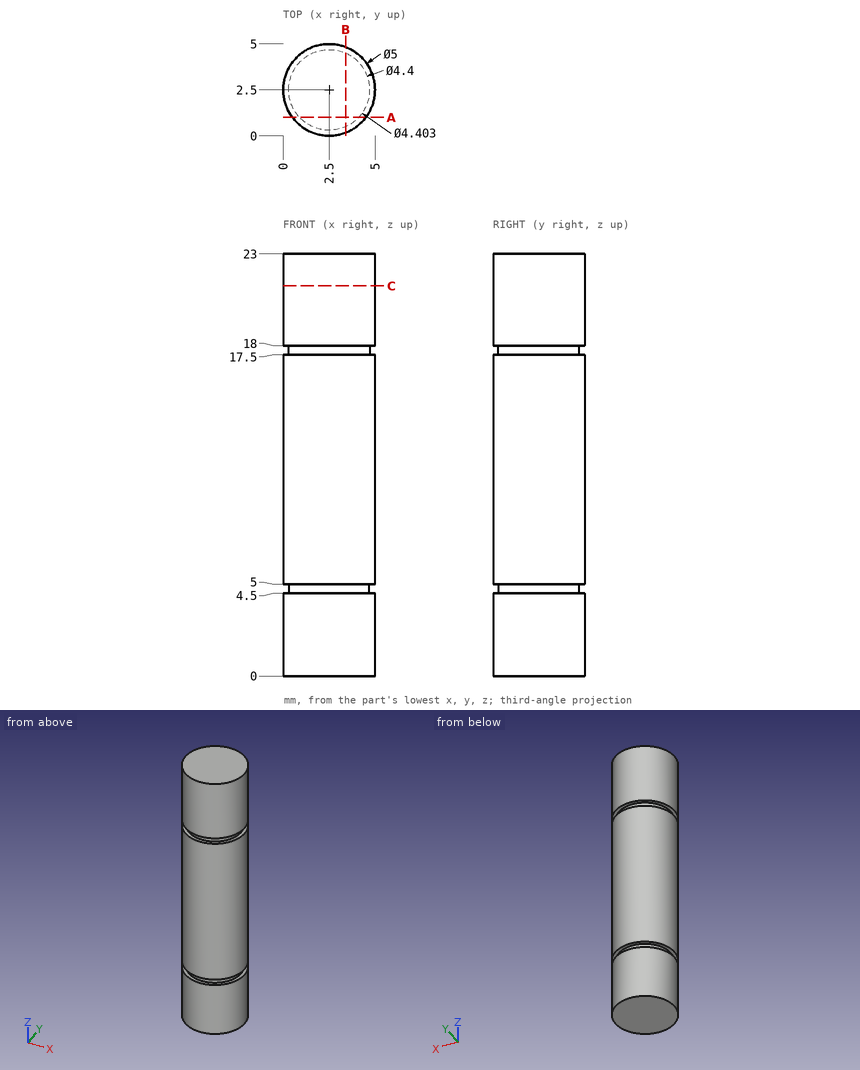
Print and shaded views of the part. All mm, measured from the part's lowest x, y and z. Round coordinates to 2 decimals unless told otherwise and drop trailing zeros. Write each loop counter-clockwise with the first axis right and the second up, starting at its lowest first coordinate (ties: lowest second). Pieces come first, ordered by that corner, then holes.
Item 1: Cut at B-B, the plane x = 3.4. Give the cut face in (y, z).
Results:
outline: (0.17, 0) - (4.83, 0) - (4.83, 4.5) - (4.51, 4.5) - (4.51, 5) - (4.83, 5) - (4.83, 17.5) - (4.51, 17.5) - (4.51, 18) - (4.83, 18) - (4.83, 23) - (0.17, 23) - (0.17, 18) - (0.49, 18) - (0.49, 17.5) - (0.17, 17.5) - (0.17, 5) - (0.49, 5) - (0.49, 4.5) - (0.17, 4.5) - close
Item 2: Cut at A-A, the plane y = 1. Give the cut face in (x, z).
Results:
outline: (0.5, 0) - (4.5, 0) - (4.5, 4.5) - (4.11, 4.5) - (4.11, 5) - (4.5, 5) - (4.5, 17.5) - (4.11, 17.5) - (4.11, 18) - (4.5, 18) - (4.5, 23) - (0.5, 23) - (0.5, 18) - (0.89, 18) - (0.89, 17.5) - (0.5, 17.5) - (0.5, 5) - (0.89, 5) - (0.89, 4.5) - (0.5, 4.5) - close
Item 3: Drop flat-ended pins along their axis: pin 1 Ø1 at (y, z) = (1.5, 8) entering from +X; pin 2 Ø1 at (y, z) = (1.5, 5.5) entering from -X; pin 3 Ø1 at (x, z) = (2, 4) entering from -Y. Give the stop position or say it passes through.
Results:
pin 1: stops at x = 4.95
pin 2: stops at x = 0.05
pin 3: stops at y = 0
Item 4: Cut at C-C, the plane z = 21.25. Give the cut face in (x, y), plus the area to 3 significant figures.
Results:
outline: circle Ø5 at (2.5, 2.5)
area: 19.6 mm2
Item 5: Probe L1, parallel to Z at x = 4.3, y = 0.8; L2, parallel to Y at x = 2.4, z = 14; L3, parallel to Y at x = 2, z = 20.5. List the from-to ranges inside material, lowest first.
Results:
L1: z = 0 to 4.5, 5 to 17.5, 18 to 23
L2: y = 0 to 5
L3: y = 0.05 to 4.95
